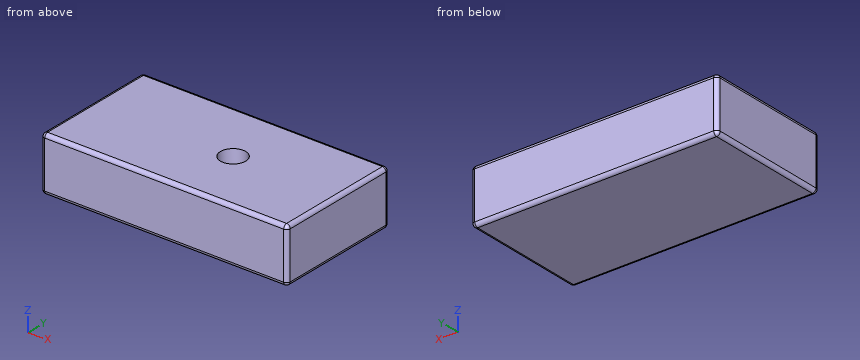
from build123d import *

# Parameters (mm, degrees)
SKETCH1_W           = 68
SKETCH1_H           = 35
BOSS_EXTRUDE1_DEPTH = 15
FILLET1_R           = 1
FILLET2_R           = 1
FILLET3_R           = 1
FILLET4_R           = 1
SKETCH2_R           = 3.5
CUT_EXTRUDE1_DEPTH  = 5


with BuildPart() as part:
    # Sketch1 → Boss-Extrude1 (new body)
    with BuildSketch(Plane.XY):
        Rectangle(SKETCH1_W, SKETCH1_H)
    extrude(amount=BOSS_EXTRUDE1_DEPTH)

    # Fillet1
    fillet1_edges = [part.edges().sort_by_distance(p)[0] for p in [
        (-34, 0, 15),
        (-34, 0, 0),
    ]]
    fillet(fillet1_edges, radius=FILLET1_R)

    # Fillet2
    fillet2_edges = [part.edges().sort_by_distance(p)[0] for p in [
        (34, 0, 15),
        (34, 0, 0),
    ]]
    fillet(fillet2_edges, radius=FILLET2_R)

    # Fillet3
    fillet3_edges = [part.edges().sort_by_distance(p)[0] for p in [
        (-34, -17.5, 7.5),
        (0, -17.5, 0),
        (0, -17.5, 15),
        (-33.707106781, -17.5, 14.707106781),
        (-33.707106781, -17.5, 0.292893219),
        (34, -17.5, 7.5),
        (33.707106781, -17.5, 14.707106781),
        (33.707106781, -17.5, 0.292893219),
    ]]
    fillet(fillet3_edges, radius=FILLET3_R)

    # Fillet4
    fillet4_edges = [part.edges().sort_by_distance(p)[0] for p in [
        (-34, 17.5, 7.5),
        (-33.707106781, 17.5, 14.707106781),
        (-33.707106781, 17.5, 0.292893219),
        (34, 17.5, 7.5),
        (0, 17.5, 0),
        (0, 17.5, 15),
        (33.707106781, 17.5, 14.707106781),
        (33.707106781, 17.5, 0.292893219),
    ]]
    fillet(fillet4_edges, radius=FILLET4_R)

    # Sketch2 → Cut-Extrude1 (cut)
    with BuildSketch(Plane.XY.offset(15)):
        with Locations((5, 0)):
            Circle(SKETCH2_R)
    extrude(amount=-CUT_EXTRUDE1_DEPTH, mode=Mode.SUBTRACT)


solid = part.part
Geometry: final body of the model. Coordinates: model frame, mm. Give positions to 0.01 mm unless a question says otherwise; leave off trailing zeros. Loops run counter-clockwise (first coordinate to the right, second up) from the corner with the lowest first, then second, coordinate; pieces in that order, holes last. Notation, with made-up numbers: M 6.5,32 L 34.5,32 A22 cw 34.5,48 Z; hole C 69,-39 d1. An arc over 180 degrees is marked long. Put each result on its own line as item: value. Start each with the question number.
1) Cut plane B-B (y = 0). Output: boundary loops of the cut face in (x, z), then the cut area to 3 significant figures.
2) Cut plane A-A (z = 12.75). Output: boundary loops of the cut face in (x, y).
3) Cut plane C-C (x = 5). Output: boundary loops of the cut face in (y, z), then the cut area to 3 significant figures.
4) Contact query for a flat-ended pin moving along its axis: pin 1 (2 mm diameter, centred on x = 6.5, y = 1.5, fed in from +Z). Output: stop coordinate, or through.
5) Ray query, line 1 along Y through (x, z) = (5, 12.25); line 2 along Y through (x, z) = (7, 14.25); line 3 along X through (y, z) = (-3, 10.5). Return the intervals inside material, ascending.
Verdict:
1. outline: M -34,1 A1 ccw -33,0 L 33,0 A1 ccw 34,1 L 34,14 A1 ccw 33,15 L 8.5,15 L 8.5,10 L 1.5,10 L 1.5,15 L -33,15 A1 ccw -34,14 Z
1. area: 984 mm2
2. outline: M -34,-16.5 A1 ccw -33,-17.5 L 33,-17.5 A1 ccw 34,-16.5 L 34,16.5 A1 ccw 33,17.5 L -33,17.5 A1 ccw -34,16.5 Z; hole C 5,0 d7
3. outline: M -17.5,1 A1 ccw -16.5,0 L 16.5,0 A1 ccw 17.5,1 L 17.5,14 A1 ccw 16.5,15 L 3.5,15 L 3.5,10 L -3.5,10 L -3.5,15 L -16.5,15 A1 ccw -17.5,14 Z
3. area: 489 mm2
4. pin 1: z = 10
5. line 1: -17.5 to -3.5, 3.5 to 17.5
5. line 2: -17.47 to -2.87, 2.87 to 17.47
5. line 3: -34 to 3.2, 6.8 to 34
